Part model, mm, in its own coordinate system. Face numbers are marked on the shaded views. A direction names the side the tool comes from. Coordinates: 2 decimals unless noted, no trailing zeros. Write each loop counter-clockwise with the first axis right and the second up, starting at its lowest first coordinate (ties: lowest second). Pieces come first, ordered by that corner, then holes. Notation, with made-up numbers: (16, 39) - (39, 39) arc R19 cw to (39, 50) - close; hole circle Ø6 at (19.5, 77.25). An arc over 180 degrees is marked (long way). Write each question's results on one line, items separated by ' | '.
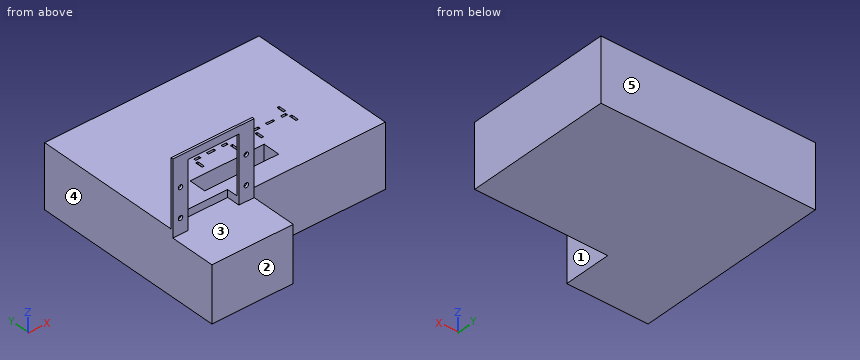
from build123d import *

# Parameters (mm, degrees)
CROQUIS1_W              = 110
CROQUIS1_H              = 65
SALIENTE_EXTRUIR1_DEPTH = 75
CROQUIS3_W              = 110
CROQUIS3_H              = 3
SALIENTE_EXTRUIR2_DEPTH = 70
CROQUIS4_R              = 3
CORTAR_EXTRUIR1_DEPTH   = 70
SALIENTE_EXTRUIR3_DEPTH = 3
CROQUIS7_W              = 290
CROQUIS7_H              = 85
SALIENTE_EXTRUIR4_DEPTH = 200
CROQUIS8_W              = 69
CROQUIS8_H              = 15
CORTAR_EXTRUIR2_DEPTH   = 10
CORTAR_EXTRUIR3_DEPTH   = 50
CROQUIS12_W             = 7
CROQUIS12_H             = 3
CROQUIS12_W_2           = 3
CROQUIS12_H_2           = 10
CROQUIS12_W_3           = 10
CORTAR_EXTRUIR4_DEPTH   = 3


with BuildPart() as part:
    # Croquis1 → Saliente-Extruir1 (new body)
    with BuildSketch(Plane.XY):
        with Locations((-30.634930344, 26.158405172)):
            Rectangle(CROQUIS1_W, CROQUIS1_H)
    extrude(amount=SALIENTE_EXTRUIR1_DEPTH)

    # Croquis3 → Saliente-Extruir2 (add)
    with BuildSketch(Plane.XY.offset(75)):
        with Locations((-30.634930344, 57.158405172)):
            Rectangle(CROQUIS3_W, CROQUIS3_H)
    extrude(amount=SALIENTE_EXTRUIR2_DEPTH)

    # Croquis4 → Cortar-Extruir1 (cut)
    with BuildSketch(Plane.XZ.offset(-55.658405172)):
        with Locations(Location((-75.134930344, 134.5, 0), (0, 0, 270))):
            Circle(CROQUIS4_R)
        with Locations(Location((-75.134930344, 95.5, 0), (0, 0, 270))):
            Circle(CROQUIS4_R)
        with Locations(Location((13.865069656, 134.5, 0), (0, 0, 270))):
            Circle(CROQUIS4_R)
        with Locations(Location((13.865069656, 95.5, 0), (0, 0, 270))):
            Circle(CROQUIS4_R)
        Polygon((-65.134930344, 134.5), (-65.134930344, 75), (3.865069656, 75), (3.865069656, 138), (3.865069656, 145), (-65.134930344, 145), align=None)
    extrude(amount=-CORTAR_EXTRUIR1_DEPTH, mode=Mode.SUBTRACT)

    # Croquis6 → Saliente-Extruir3 (add)
    with BuildSketch(Plane(origin=(0, 58.658405172, 0), x_dir=(1, 0, 0), z_dir=(0, 1, 0))):
        Polygon((-85.634930344, -145), (-85.634930344, -175), (24.365069656, -175), (24.365069656, -145), (3.865069656, -145), (3.865069656, -165), (-65.134930344, -165), (-65.134930344, -145), align=None)
    extrude(amount=-SALIENTE_EXTRUIR3_DEPTH)

    # Croquis7 → Saliente-Extruir4 (add)
    with BuildSketch(Plane(origin=(0, 58.658405172, 0), x_dir=(1, 0, 0), z_dir=(0, 1, 0))):
        with Locations((59.365069656, -42.5)):
            Rectangle(CROQUIS7_W, CROQUIS7_H)
    extrude(amount=SALIENTE_EXTRUIR4_DEPTH)

    # Croquis8 → Cortar-Extruir2 (cut)
    with BuildSketch(Plane.XY.offset(85)):
        with Locations((-30.634930344, 66.158405172)):
            Rectangle(CROQUIS8_W, CROQUIS8_H)
    extrude(amount=-CORTAR_EXTRUIR2_DEPTH, mode=Mode.SUBTRACT)

    # Croquis10 → Cortar-Extruir3 (cut)
    with BuildSketch(Plane.XY.offset(85)):
        Polygon((-0.634930344, 87.0941562), (-15.634930344, 87.0941562), (-15.634930344, 110.0941562), (-0.634930344, 110.0941562), (69.365069656, 110.0941562), (84.365069656, 110.0941562), (84.365069656, 87.0941562), (69.365069656, 87.0941562), align=None)
    extrude(amount=-CORTAR_EXTRUIR3_DEPTH, mode=Mode.SUBTRACT)

    # Croquis12 → Cortar-Extruir4 (cut)
    with BuildSketch(Plane.XY.offset(85)):
        with Locations((15.865069656, 135.5941562)):
            Rectangle(CROQUIS12_W, CROQUIS12_H)
        with Locations((10.865069656, 125.5941562)):
            Rectangle(CROQUIS12_W_2, CROQUIS12_H_2)
        with Locations((57.865069656, 145.5941562)):
            Rectangle(CROQUIS12_W_2, CROQUIS12_H_2)
        with Locations((57.865069656, 125.5941562)):
            Rectangle(CROQUIS12_W_2, CROQUIS12_H_2)
        with Locations((52.865069656, 135.5941562)):
            Rectangle(CROQUIS12_W, CROQUIS12_H)
        with Locations((10.865069656, 145.5941562)):
            Rectangle(CROQUIS12_W_2, CROQUIS12_H_2)
        with Locations((34.365069656, 135.5941562)):
            Rectangle(CROQUIS12_W_3, CROQUIS12_H)
        with Locations((114.365069656, 135.5941562)):
            Rectangle(CROQUIS12_W_3, CROQUIS12_H)
        with Locations((132.865069656, 135.5941562)):
            Rectangle(CROQUIS12_W, CROQUIS12_H)
        with Locations((90.865069656, 145.5941562)):
            Rectangle(CROQUIS12_W_2, CROQUIS12_H_2)
        with Locations((90.865069656, 125.5941562)):
            Rectangle(CROQUIS12_W_2, CROQUIS12_H_2)
        with Locations((95.865069656, 135.5941562)):
            Rectangle(CROQUIS12_W, CROQUIS12_H)
        with Locations((137.865069656, 145.5941562)):
            Rectangle(CROQUIS12_W_2, CROQUIS12_H_2)
        with Locations((137.865069656, 125.5941562)):
            Rectangle(CROQUIS12_W_2, CROQUIS12_H_2)
    extrude(amount=-CORTAR_EXTRUIR4_DEPTH, mode=Mode.SUBTRACT)


solid = part.part
(1) Wall check: line 1 (X direction, y = 56.4, z = 134.5); line 2 (X direction, y = 57, z = 134); line 3 (Y direction, x = 0, z = 59). Give the ranges that are in metal, low to high. Write a range as from..to.
Return value:
line 1: x = -85.63..-78.13, -72.13..-65.13, 3.87..10.87, 16.87..24.37 | line 2: x = -85.63..-78.09, -72.18..-65.13, 3.87..10.91, 16.82..24.37 | line 3: y = -6.34..87.09, 110.09..258.66
(2) 3-axis set-ups, long thin cutter, end or side, ignore diameter. For the marked faces 1 and 2: which of +Z, -Z, +X, -X, +Y, -Y reach the whole face in a straight line?
Return value:
face 1: +Z, -Z, +X, -Y | face 2: +Z, -Z, +X, -X, -Y
(3) Flat gauge pins, fed straight in: P1, Ø1, axis at x = -48.5, y = 146.5, coming from the +Z side; P2, Ø3.5, axis at x = 138, z = 84, coming from the -Y side; P3, Ø2.5, axis at x = 16.5, y = 135.5, coming from the +Z side; P4, Ø5.5, axis at x = 13.87, z = 95.5, coming from the +Y side. Where does each tip first touch, or does it go through?
Return value:
P1: stops at z = 85 | P2: stops at y = 58.66 | P3: stops at z = 82 | P4: passes through
(4) Two-plate mould, pull along X, no slides. Class the marked faces 3, 4 and 5: released by +X, released by -X, zero draft, split by the parting line, or undercut.
Return value:
face 3: undercut | face 4: released by -X | face 5: zero draft
(5) Saw through at C-C on z = 53. Write the cut outline in (x, y).
Return value:
outline: (-85.63, -6.34) - (24.37, -6.34) - (24.37, 58.66) - (204.37, 58.66) - (204.37, 258.66) - (-85.63, 258.66) - close; hole (-15.63, 87.09) - (84.37, 87.09) - (84.37, 110.09) - (-15.63, 110.09) - close
(6) Saw through at A-A on z = 142.5. Write the cut outline in (x, y), then the cut area to 3 significant figures.
Return value:
outline: (-85.63, 55.66) - (-65.13, 55.66) - (-65.13, 58.66) - (-85.63, 58.66) - close; (3.87, 55.66) - (24.37, 55.66) - (24.37, 58.66) - (3.87, 58.66) - close | area: 123 mm^2
(7) Saw through at B-B on y = 146. Write the cut outline in (x, z), then the cut area to 3 significant figures.
Return value:
outline: (-85.63, 0) - (204.37, 0) - (204.37, 85) - (139.37, 85) - (139.37, 82) - (136.37, 82) - (136.37, 85) - (92.37, 85) - (92.37, 82) - (89.37, 82) - (89.37, 85) - (59.37, 85) - (59.37, 82) - (56.37, 82) - (56.37, 85) - (12.37, 85) - (12.37, 82) - (9.37, 82) - (9.37, 85) - (-85.63, 85) - close | area: 24,600 mm^2
